```python
from build123d import *

# Parameters (mm, degrees)
F0_R     = 20.066
F1_DEPTH = 29.21
F2_R     = 13.97
F3_DEPTH = 7.62
F5_D     = 10.3


with BuildPart() as f1:
    # F0 (on Front) → F1 (new body)
    with BuildSketch(Plane.XZ):
        Circle(F0_R)
    extrude(amount=F1_DEPTH)

    # F2 (on face) → F3 (cut)
    with BuildSketch(Plane.XZ.offset(29.21)):
        Circle(F2_R)
    extrude(amount=-F3_DEPTH, mode=Mode.SUBTRACT)

    # F5 (through all)
    with Locations(Plane(origin=(0, 0, 0), x_dir=(-1, 0, 0), z_dir=(0, 1, 0))):
        with Locations((0, 0)):
            Hole(F5_D / 2)


solid = f1.part
```
CAD build for the part. Positions are in the model's coordinates, mm. A direction names the side the tool comes from. Coordinates: 2 decimals unless noted, no trailing zeros. Order: outer loops, then holes, each group sorted by start corner. A loop starts at its lowest first (then second) coordinate and runs counter-clockwise, first axis right, second up. Notation, with made-up numbers: (3, 26) - (44, 26) arc R31 ccw to (44, 56) - close; hole circle Ø8 at (41.25, -23.5). An arc over 180 degrees is marked (long way). Use a Markdown table: item, result. Add a question column.
(1) Saw through at A-A (z = 0). Give the cut face in (x, y), then the cut area to 3 significant figures.
(2) Saw through at C-C (x = -13). Give the cut face in (y, z), then the cut area to 3 significant figures.
(3) Drill centre lines: line 1 along Z through (x, y) = (0, -5); line 2 along Z through (x, y) = (0, -24); line 3 along X through (y, z) = (-23.75, 0.5). Where is each one in solid material? Low to high. Write a range as [from, to].
(4) Which spindle directions (+Z, -Z, +X, -X, +Y, -Y) get a long thin tool onto all of the face, cutting with end or side? Do faces 1 (the face through (6, -21.59, 0)), 2 (the face through (4.91, -10.95, 1.55)). Say none if no direction does.
(5) Flat gauge pins, fed straight in: pin 1 (5 mm diameter, centred on y = -10.5, z = -16, fed in from +X); pin 2 (1.5 mm diameter, centred on y = -18, z = -12.5, fed in from -X); pin 3 (12 mm diameter, centred on y = -9.5, z = -12.5, fed in from -X); pin 4 (9.5 mm diameter, centred on x = 0, z = 0, fed in from -Y). Where does each tip first touch, or does it go through?
(6) Pull direction X, two halves, no side cores. Call faces 3 (the face through (-4.3, -14.4, -19.6)), 4 (the face through (4, 0, -4)), 5 (the face through (-1.82, -25.45, 13.85)): +X half, -X half, draft (parallel to the pull), parting line (faces both ways), or undercut.
(7) Saw through at B-B (x = 0). Give the cut face in (y, z), then the cut area to 3 significant figures.
(8) Saw through at D-D (y = -10.5). Give the cut face in (x, z), then the cut area to 3 significant figures.
Solved:
| question | item | result |
|---|---|---|
| 1 | outline | (-20.07, -29.21) - (-13.97, -29.21) - (-13.97, -21.59) - (-5.15, -21.59) - (-5.15, 0) - (-20.07, 0) - close; (5.15, -21.59) - (13.97, -21.59) - (13.97, -29.21) - (20.07, -29.21) - (20.07, 0) - (5.15, 0) - close |
| 1 | area | 737 mm² |
| 2 | outline | (-29.21, -15.29) - (0, -15.29) - (0, 15.29) - (-29.21, 15.29) - (-29.21, 5.11) - (-21.59, 5.11) - (-21.59, -5.11) - (-29.21, -5.11) - close |
| 2 | area | 815 mm² |
| 3 | line 1 | z = [-20.07, -5.15], [5.15, 20.07] |
| 3 | line 2 | z = [-20.07, -13.97], [13.97, 20.07] |
| 3 | line 3 | x = [-20.06, -13.96], [13.96, 20.06] |
| 4 | face 1 | -Y |
| 4 | face 2 | +Y, -Y |
| 5 | pin 1 | stops at x = 14.85 |
| 5 | pin 2 | stops at x = -16.27 |
| 5 | pin 3 | stops at x = -18.98 |
| 5 | pin 4 | passes through |
| 6 | face 3 | parting line |
| 6 | face 4 | draft |
| 6 | face 5 | undercut |
| 7 | outline | (-29.21, -20.07) - (0, -20.07) - (0, -5.15) - (-21.59, -5.15) - (-21.59, -13.97) - (-29.21, -13.97) - close; (-29.21, 13.97) - (-21.59, 13.97) - (-21.59, 5.15) - (0, 5.15) - (0, 20.07) - (-29.21, 20.07) - close |
| 7 | area | 737 mm² |
| 8 | outline | circle Ø40.13 at (0, 0); hole circle Ø10.3 at (0, 0) |
| 8 | area | 1,180 mm² |
